from build123d import *

# Parameters (mm, degrees)
ESBO_O2_R             = 11
CORTE_EXTRUS_O1_DEPTH = 10
ESBO_O7_R             = 1.25
CHANFRO1_SIZE         = 1.5


with BuildPart() as part:
    # Esboço1 → Revolução1 (revolve)
    with BuildSketch(Plane.XY):
        Polygon((0, 0), (11, 0), (11, 3.5), (4, 3.5), (4, 132.66), (0, 132.66), align=None)
    revolve(axis=Axis((0, 132.66, 0), (0, -1, 0)))

    # Esboço2 → Corte-extrusão1 (cut)
    with BuildSketch(Plane.XZ):
        Circle(ESBO_O2_R)
        with BuildLine():
            ThreePointArc((7.5, -0.1), (6.064823228, -3.564823228), (2.6, -5))
            Line((2.6, -5), (-2.6, -5))
            ThreePointArc((-2.6, -5), (-6.064823228, -3.564823228), (-7.5, -0.1))
            Line((-7.5, -0.1), (-7.5, 0.1))
            ThreePointArc((-7.5, 0.1), (-6.064823228, 3.564823228), (-2.6, 5))
            Line((-2.6, 5), (2.6, 5))
            ThreePointArc((2.6, 5), (6.064823228, 3.564823228), (7.5, 0.1))
            Line((7.5, 0.1), (7.5, -0.1))
        make_face(mode=Mode.SUBTRACT)
    extrude(amount=-CORTE_EXTRUS_O1_DEPTH, mode=Mode.SUBTRACT)

    # Varredura1: sweep along a path in Esboço9
    with BuildLine(Plane.XY) as varredura1_path:
        ThreePointArc((-6, 0), (0, -6), (6, 0))
    # Esboço7 → Varredura1 (sweep)
    with BuildSketch(Plane(origin=(0, 0, 0), x_dir=(-1, 0, 0), z_dir=(0, -1, 0))):
        with Locations((6, 0)):
            Circle(ESBO_O7_R)
    sweep(path=varredura1_path.line)

    # Chanfro1
    chanfro1_edges = [part.edges().sort_by_distance(p)[0] for p in [
        (-4, 132.66, 0),
    ]]
    chamfer(chanfro1_edges, length=CHANFRO1_SIZE)


solid = part.part
For this review, take the finished solid that the model builds, in its own axes (mm). A direction names the side the tool comes from. Give positions to 0.01 mm unless a question says otherwise; leave off trailing zeros. Loops run counter-clockwise (first coordinate to the right, second up) from the corner with the lowest first, then second, coordinate; pieces in that order, holes last. Notation, with made-up numbers: M 7,-17.5 L 14,-17.5 A22 ccw 14,-3.5 Z; hole C 25.5,-34 d8. An arc over 180 degrees is marked long. Answer as a JSON object with one key per item and string values. Group by question number.
Q1. Add section B-B on y = 99. Give the boundary of the cut face in (x, z).
Q2. Insertion check: P1, Ø2, axis at x = -4.5, z = 3, coming from the -Y side; P2, Ø6, axis at x = 4.5, y = 32.5, coming from the +Z side; P3, Ø1.5, axis at y = 85, z = -0.5, coming from the -X side. Each pin has a flat end and moves straight along its axis. Give the tip position at first contact, or say it passes through.
Q3. Tool access review of faces 4 (the cylindrical face through (-0.867, 68.224, -3.905)), 5 (the flat face through (0, 2, -5)): name each direction out of +Z, -Z, +X, -X, +Y, -Y from which nothing blocks a thin tool from reaching the whole face with its end or side.
Q4. For probe 1 along Y at (x, z) = (1.5, 3.75); probe 2 along Y at (x, z) = (2.5, 0.25); probe 3 along X at (y, z) = (1.5, -1), list the stretches that pass through material, from the lowest coordinate up. Write a range as [from, to].
Q5. Mouldability with a two-part tool opening along Y and no side actions: class faces 1 (the flat face through (0, 132.66, 0)), 2 (the flat face through (0, 0, 0)), 3 (the cylindrical face through (-6.03, 1.73, -3.6)) as +Y half, -Y half, draft (parallel to the pull), parting line (faces both ways), or undercut.
Q6. Add section A-A on x = 0. Give the boundary of the cut face in (y, z).
Checked values:
{
 "1": {"outline": "C 0,0 d8"},
 "2": {"P1": "y = 0", "P2": "z = 3.71", "P3": "x = -4"},
 "3": {"face 4": "+Y", "face 5": "-Z, +X, -X, +Y, -Y"},
 "4": {"probe 1": "[0, 3.5]", "probe 2": "[-6.78, -4.07], [0, 132.65]", "probe 3": "[-7.42, 7.42]"},
 "5": {"face 1": "+Y half", "face 2": "undercut", "face 3": "draft"},
 "6": {"outline": "C -6,0 d2.5; M 0,-5 L 3.5,-5 L 3.5,-4 L 131.16,-4 L 132.66,-2.5 L 132.66,2.5 L 131.16,4 L 3.5,4 L 3.5,5 L 0,5 Z"}
}
